Autodesk Inventor part; units mm, degrees
ref_plane "YZ Plane" through (0, 0, 0) normal (1, 0, 0) x (0, 1, 0)
ref_plane "XZ Plane" through (0, 0, 0) normal (0, 1, 0) x (-1, 0, 0)
ref_plane "XY Plane" through (0, 0, 0) normal (0, 0, 1) x (1, 0, 0)
sketch "Sketch1" plane through (0, 0, 0) normal (0, 0, 1) x (1, 0, 0)
  line L0 (-8.5, -205) -> (8.5, -205)
  line L1 (8.5, -205) -> (8.5, 205)
  line L2 (8.5, 205) -> (-8.5, 205)
  line L3 (-8.5, 205) -> (-8.5, -205)
  line L4 (-8.5, -205) -> (8.5, 205) construction
  line L5 (8.5, -205) -> (-8.5, 205) construction
  line L6 (-2.4, 211) -> (2.4, 211)
  line L7 (2.4, 211) -> (2.4, 205)
  line L8 (2.4, 205) -> (-2.4, 205)
  line L9 (-2.4, 205) -> (-2.4, 211)
  line L10 (-2.4, 211) -> (2.4, 205) construction
  line L11 (2.4, 211) -> (-2.4, 205) construction
  line L12 (-8.5, 0) -> (8.5, 0)
  line L13 (-2.4, -211) -> (2.4, -211)
  line L14 (2.4, -211) -> (2.4, -205)
  line L15 (2.4, -205) -> (-2.4, -205)
  line L16 (-2.4, -205) -> (-2.4, -211)
  line L17 (-2.4, -211) -> (2.4, -205) construction
  line L18 (2.4, -211) -> (-2.4, -205) construction
  point P0 (0, 0)
  point P1 (0, 208)
  point P2 (0, 205)
  point P3 (0, 205)
  point P4 (0, -208)
  point P5 (0, -205)
  point P6 (0, -205)
  dimension "d0" = 17
  dimension "d1" = 410
  dimension "d2" = 4.8
  dimension "d3" = 6
extrude "Plate1" add sketch "Sketch1" along normal mid plane 3
equation "\"d4\" = Thickness"
equation "\"BendRadius\" = Thickness"
equation "\"BendReliefWidth\" = Thickness"
equation "\"BendReliefDepth\" = 0.5 * Thickness"
equation "\"CornerReliefSize\" = 4 * Thickness"
equation "\"MinimumRemnant\" = 2 * Thickness"
equation "\"TransitionRadius\" = BendRadius"
equation "\"JacobiRadiusSize\" = BendRadius"
equation "\"GapSize\" = Thickness"
properties part number "Path Holder"
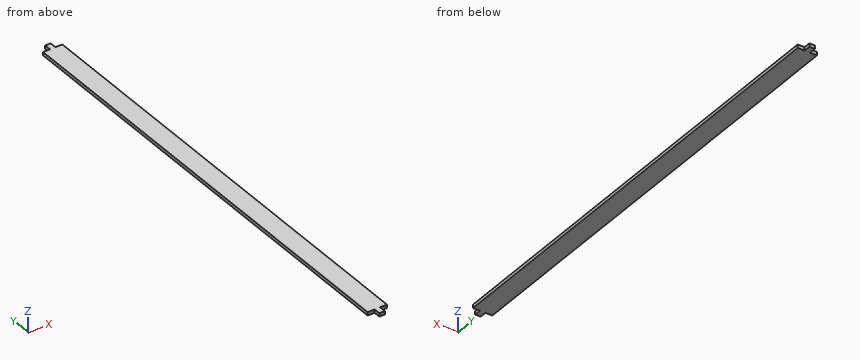
Geometry check sheet. Reference: the model listing, model coordinates, mm. Give positions to 0.01 mm unless a question says otherwise; leave off trailing zeros. Loops run counter-clockwise (first coordinate to the right, second up) from the corner with the lowest first, then second, coordinate; pieces in that order, holes last. Notation, with made-up numbers: (50.5, 75) - (63.5, 75) arc R27 ccw to (63.5, 95) - close; hole circle Ø6 at (-26.75, 81). An arc over 180 degrees is marked (long way). Use CSV: the item, a comma, the result in double quotes. Start each with the question number.
Q1. Section check A-A, the plane z = -0.2. Record the cut outline in (x, y), and give its area (3 significant figures).
Q2. Section check B-B, the plane x = -5.25. Record the cut outline in (y, z).
Q3. Go/stop test with flat-tipped pins: pin 1 Ø0.9 at (y, z) = (208.5, 0.5) entering from +X; pin 2 Ø1.5 at (x, z) = (6.5, -0.5) entering from -Y. Record where each tip stops, or that it passes through.
Q4. Scan line: probe 1 along Y at (x, z) = (6.5, -0.6). Record every from-to range of solid material in increasing order. Write a range as from..to.
Findings below:
1,outline,"(-8.5, -205) - (-2.4, -205) - (-2.4, -211) - (2.4, -211) - (2.4, -205) - (8.5, -205) - (8.5, 205) - (2.4, 205) - (2.4, 211) - (-2.4, 211) - (-2.4, 205) - (-8.5, 205) - close"
1,area,"7,030 mm^2"
2,outline,"(-205, -1.5) - (205, -1.5) - (205, 1.5) - (-205, 1.5) - close"
3,pin 1,"stops at x = 2.4"
3,pin 2,"stops at y = -205"
4,probe 1,"y = -205..205"
